Can you work these out from the model? Positions are in its coordinate system, mm. A direction names the side the tool comes from. Coordinates: 2 decimals unless noted, no trailing zeros. Order: outer loops, then holes, each group sorted by start corner. A loop starts at its lowest first (then second) coordinate and runs counter-clockwise, first axis right, second up. Notation, with made-up numbers: (77.25, -36) -> (90.25, -36) arc R14 ccw to (90.25, -21) -> close; hole circle Ø4 at (36.5, 86.25). An arc over 180 degrees is marked (long way). Answer as a JSON object with one key per item and string values. Group by question number.
(1) If we mould it in two halves opening along Z, with no side actions, what happens to faces 1 (the flat face through (0, 2, -50)), 2 (the flat face through (-11.25, 2, -1)), 3 (the cylindrical face through (-8.24, 2.02, 47.15)), 4 (the cylindrical face through (-0.46, 2.08, -47.47))? For each: pulls with the +Z half, pulls with the -Z half, needs draft (parallel to the pull), parting line crosses it, or undercut.
(2) For pin 1 (1 mm diameter, centred on x = -3, y = 2.5, fed in from -Z); pin 2 (3 mm diameter, centred on x = 0.5, z = -32, fed in from +Y), each with a flat end and sliding along its axis, tell me the tip position at first contact or that it passes through.
(3) I want a section at A-A, the plane x = 0. List the corners of the cut face in (y, z) for me, plus the area to 3 significant figures.
(4) Which directions (+Z, -Z, +X, -X, +Y, -Y) give clear straight access to the entire face, cutting with the end or side of a thin tool? Please do faces 5 (the cylindrical face through (0, 3.6, -26.5)), 6 (the flat face through (0, 4.1, 1)).
(5) I need wall thicknesses on line 1 (Z direction, x = 0, y = 1.3); line 2 (Z direction, x = 0, y = 3.8); line 3 (X direction, y = 2.9, z = -44). Which ranges of each line are inside material? Lowest first, please.
(6) I want a section at B-B, the plane z = -44. List the corners of the cut face in (x, y) for me, plus the area to 3 significant figures.
(7) I want a section at C-C, the plane y = 1.85. List the corners of the cut face in (x, z) for me.
(8) I want a section at D-D, the plane z = -27.5. List the corners of the cut face in (x, y) for me, plus the area to 3 significant figures.
Autodesk Inventor part; units mm, degrees
ref_plane "YZ Plane" through (0, 0, 0) normal (1, 0, 0) x (0, 1, 0)
ref_plane "XZ Plane" through (0, 0, 0) normal (0, 1, 0) x (-1, 0, 0)
ref_plane "XY Plane" through (0, 0, 0) normal (0, 0, 1) x (1, 0, 0)
sketch "Szkic1" plane through (0, 0, 0) normal (0, 1, 0) x (-1, 0, 0)
  line L0 (1.25, 50) -> (-1.25, 50)
  line L1 (-11.25, 40) -> (-11.25, -40)
  line L2 (-1.25, -50) -> (1.25, -50)
  line L3 (11.25, -40) -> (11.25, 40)
  line L4 (11.25, 50) -> (-11.25, -50)
  line L5 (11.25, -50) -> (-11.25, 50)
  arc A0 (11.25, 40) -> (1.25, 50) centre (1.25, 40) ccw
  arc A1 (-1.25, 50) -> (-11.25, 40) centre (-1.25, 40) ccw
  arc A2 (1.25, -50) -> (11.25, -40) centre (1.25, -40) ccw
  arc A3 (-11.25, -40) -> (-1.25, -50) centre (-1.25, -40) ccw
  point P0 (0, 0)
  point P1 (0, 0)
  dimension "d0" = 22.5
  dimension "d1" = 100
  dimension "d2" = 10
extrude "Wyciągnięcie proste1" add sketch "Szkic1" along normal blind 4.1
sketch "Szkic2" plane through (0, 4.1, 0) normal (0, 1, 0) x (1, 0, 0)
  circle A0 centre (0, 44) radius 3.5
  line L0 (1.25, 50) -> (-1.25, 50)
  point P0 (0, 0)
  point P1 (0, 50)
  dimension "d5" = 7
  dimension "d14" = 6
extrude "Wyciągnięcie proste2" cut sketch "Szkic2" against normal blind 8
sketch "Szkic3" plane through (0, 4.1, 0) normal (0, 1, 0) x (1, 0, 0)
  line L0 (0, 47.5) -> (0, 28.5)
  arc A0 (-2, 28.5) -> (2, 28.5) centre (0, 28.5) ccw
  line L1 (-2.75, 41.8349) -> (0, 41.8349)
  line L2 (1.25, 50) -> (-1.25, 50)
  line L3 (-2, 28.5) -> (-2.75, 41.8349)
  line L4 (2, 28.5) -> (2.75, 41.8349)
  line L5 (0, 41.8349) -> (2.75, 41.8349)
  circle A1 centre (0, 44) radius 3.5
  point P0 (0, 0)
  point P1 (0, 50)
  dimension "d8" = 19
  dimension "d10" = 5.5
extrude "Wyciągnięcie proste3" cut sketch "Szkic3" against normal blind 1.1 contours L5 A1 L0 | L0 A1 L1 | A1 L4 A0 L3 picked at (1.6483, 41.6479) picked at (-1.6483, 41.6479)
sketch "Szkic4" plane through (0, 4.1, 0) normal (0, 1, 0) x (1, 0, 0)
  circle A0 centre (0, -45) radius 3.5
  line L0 (-1.25, -50) -> (1.25, -50)
  point P0 (0, 0)
  point P1 (0, -50)
  dimension "d15" = 7
  dimension "d16" = 5
extrude "Wyciągnięcie proste4" cut sketch "Szkic4" against normal blind 10
properties part number "arm_big_part"
Computed values:
{
 "1": {"face 1": "pulls with the -Z half", "face 2": "needs draft", "face 3": "pulls with the +Z half", "face 4": "undercut"},
 "2": {"pin 1": "stops at z = -49.92", "pin 2": "stops at y = 3"},
 "3": {"outline": "(0, -50) -> (4.1, -50) -> (4.1, -47.5) -> (0, -47.5) -> close; (0, -40.5) -> (3, -40.5) -> (3, -26.5) -> (4.1, -26.5) -> (4.1, 41.5) -> (0, 41.5) -> close; (0, 48.5) -> (4.1, 48.5) -> (4.1, 50) -> (0, 50) -> close", "area": "337 mm2"},
 "4": {"face 5": "+Y", "face 6": "+Z, -Z, +X, -X, +Y"},
 "5": {"line 1": "z = -50 to -47.5, -40.5 to 41.5, 48.5 to 50", "line 2": "z = -50 to -47.5, -26.5 to 41.5, 48.5 to 50", "line 3": "x = -10.42 to -3.5, 3.5 to 10.42"},
 "6": {"outline": "(-10.42, 0) -> (-3.5, 0) -> (-3.5, 4.1) -> (-10.42, 4.1) -> close; (3.5, 0) -> (10.42, 0) -> (10.42, 4.1) -> (3.5, 4.1) -> close", "area": "56.7 mm2"},
 "7": {"outline": "(-11.25, -40) arc R10 ccw to (-1.25, -50) -> (1.25, -50) arc R10 ccw to (11.25, -40) -> (11.25, 40) arc R10 ccw to (1.25, 50) -> (-1.25, 50) arc R10 ccw to (-11.25, 40) -> close; hole circle Ø7 at (0, -44); hole circle Ø7 at (0, 45)"},
 "8": {"outline": "(-11.25, 0) -> (11.25, 0) -> (11.25, 4.1) -> (1.73, 4.1) -> (1.73, 3) -> (-1.73, 3) -> (-1.73, 4.1) -> (-11.25, 4.1) -> close", "area": "88.4 mm2"}
}
